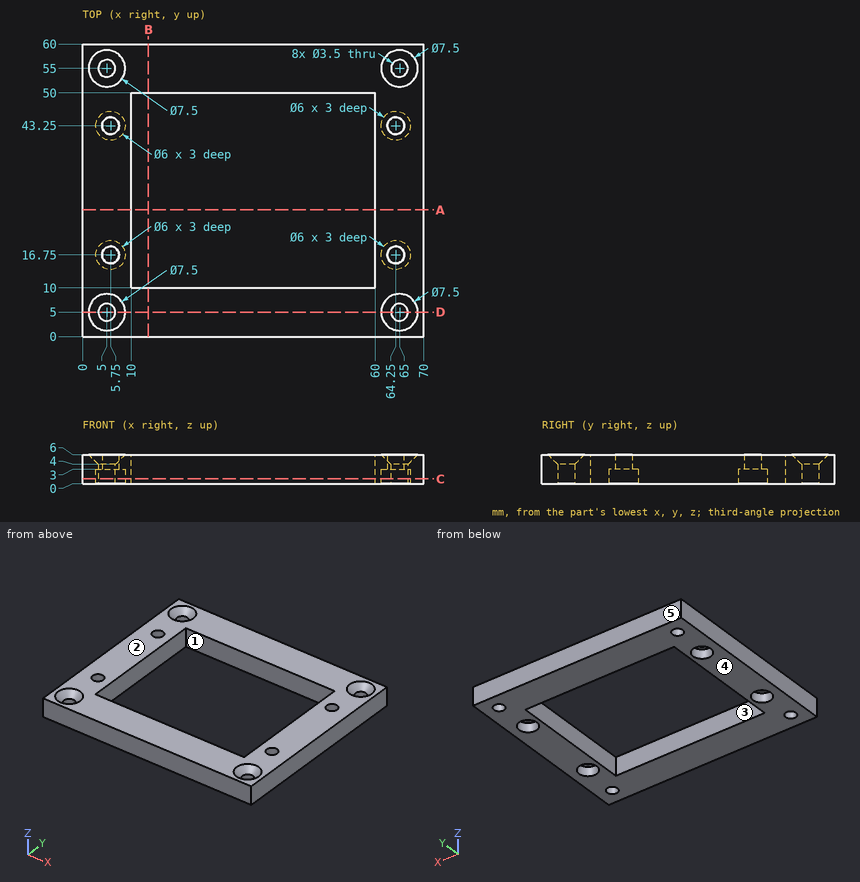
Study the drawing (mm; zero at the part's minimum x, y, z) and answer. A direction names the side the tool comes from. Coordinates: 2 decimals unless noted, no trailing zeros. Write each loop counter-clockwise with the first axis right and the second up, starting at its lowest first coordinate (ties: lowest second). Pieces come first, ordered by that corner, then holes.
Q1. Which of the six approach directions +Z, -Z, +X, -X, +Y, -Y give full straight-line access (tool end or side, diameter ignored) to the marked faces 1 and 2?
Q2. Each of these flat-tipped pins is pushed along its axis until it touches: pin 1 Ø4 at (x, y) = (64.25, 43.25) entering from -Z; pin 2 Ø3 at (x, y) = (5.75, 43.25) entering from +Z. Where does it stop, or does it pass through?
Q3. A cutting plane is placed at C-C, the plane z = 1.05. State how many separate pieces and enclosed holes the cut face has, then the cut area to 3 significant figures.
Q4. A cutting plane is placed at B-B, the plane x = 13.5. Give the vertices of the cut face in (y, z), then the cut area to 3 significant figures.
Q5. A cutting plane is placed at D-D, the plane y = 5. Give the vertices of the cut face in (x, z), then the cut area to 3 significant figures.
Q6. Find the intervals of material crossed by line 1 (X direction, y = 17, z = 3.7); line 2 (Y direction, x = 43, z = 1.25); line 3 (Y direction, x = 5.75, z = 1.6), in increasing order.
Q7. Determine the mould class of the marked faces 3, 4 and 5 for opening direction Y: released by +Y, released by -Y, zero draft, split by the parting line, or undercut.
Q8. A cutting plane is placed at A-A, the plane y = 26. Give the vertices of the cut face in (x, z), then the cut area to 3 significant figures.
Findings below:
1. face 1: +Z, -Z
1. face 2: +Z, +X, -X, +Y, -Y
2. pin 1: stops at z = 3
2. pin 2: passes through
3. separate pieces: 1
3. enclosed holes: 9
3. area: 2,050 mm2
4. outline: (0, 0) - (10, 0) - (10, 6) - (0, 6) - close; (50, 0) - (60, 0) - (60, 6) - (50, 6) - close
4. area: 120 mm2
5. outline: (0, 0) - (3.25, 0) - (3.25, 4) - (1.25, 6) - (0, 6) - close; (6.75, 0) - (63.25, 0) - (63.25, 4) - (61.25, 6) - (8.75, 6) - (6.75, 4) - close; (66.75, 0) - (70, 0) - (70, 6) - (68.75, 6) - (66.75, 4) - close
5. area: 370 mm2
6. line 1: x = 0 to 4.02, 7.48 to 10, 60 to 62.52, 65.98 to 70
6. line 2: y = 0 to 10, 50 to 60
6. line 3: y = 0 to 3.42, 6.58 to 13.75, 19.75 to 40.25, 46.25 to 53.42, 56.58 to 60
7. face 3: undercut
7. face 4: zero draft
7. face 5: released by +Y
8. outline: (0, 0) - (10, 0) - (10, 6) - (0, 6) - close; (60, 0) - (70, 0) - (70, 6) - (60, 6) - close
8. area: 120 mm2
